Check sheet for the modelled part. Datum: model origin and axes. Units: mm. A direction names the side the tool comes from. Round coordinates to 2 decimals unless told otherwise and drop trailing zeros. Order: outer loops, then holes, each group sorted by start corner. A loop starts at its lowest first (then second) coordinate and runs counter-clockwise, first axis right, second up.
```python
from build123d import *

# Parameters (mm, degrees)
SKETCH1_W           = 5
SKETCH1_H           = 3.7
BOSS_EXTRUDE1_DEPTH = 400
SKETCH2_R           = 1.75
CUT_EXTRUDE1_DEPTH  = 2
SKETCH3_R           = 1
CUT_EXTRUDE2_DEPTH  = 401.036248358
CUT_EXTRUDE3_DEPTH  = 401.048359577
SKETCH5_W           = 10.325646163
SKETCH5_H           = 6.55225139
CUT_EXTRUDE4_DEPTH  = 200


with BuildPart() as part:
    # Sketch1 → Boss-Extrude1 (new body)
    with BuildSketch(Plane.XY):
        with Locations((2.5, 1.85)):
            Rectangle(SKETCH1_W, SKETCH1_H)
    extrude(amount=-BOSS_EXTRUDE1_DEPTH)

    # Sketch2 → Cut-Extrude1 (cut)
    with BuildSketch(Plane(origin=(0, 3.7, 0), x_dir=(1, 0, 0), z_dir=(0, 1, 0))):
        with Locations(Location((2.5, 5, 0), (0, 0, 270))):
            Circle(SKETCH2_R)
        with Locations(Location((2.5, 20, 0), (0, 0, 270))):
            Circle(SKETCH2_R)
        with Locations(Location((2.5, 35, 0), (0, 0, 270))):
            Circle(SKETCH2_R)
        with Locations(Location((2.5, 50, 0), (0, 0, 270))):
            Circle(SKETCH2_R)
        with Locations(Location((2.5, 65, 0), (0, 0, 270))):
            Circle(SKETCH2_R)
        with Locations(Location((2.5, 80, 0), (0, 0, 270))):
            Circle(SKETCH2_R)
        with Locations(Location((2.5, 95, 0), (0, 0, 270))):
            Circle(SKETCH2_R)
        with Locations(Location((2.5, 110, 0), (0, 0, 270))):
            Circle(SKETCH2_R)
        with Locations(Location((2.5, 125, 0), (0, 0, 270))):
            Circle(SKETCH2_R)
        with Locations(Location((2.5, 140, 0), (0, 0, 270))):
            Circle(SKETCH2_R)
        with Locations(Location((2.5, 155, 0), (0, 0, 270))):
            Circle(SKETCH2_R)
        with Locations(Location((2.5, 170, 0), (0, 0, 270))):
            Circle(SKETCH2_R)
        with Locations(Location((2.5, 185, 0), (0, 0, 270))):
            Circle(SKETCH2_R)
        with Locations(Location((2.5, 200, 0), (0, 0, 270))):
            Circle(SKETCH2_R)
        with Locations(Location((2.5, 215, 0), (0, 0, 270))):
            Circle(SKETCH2_R)
        with Locations(Location((2.5, 230, 0), (0, 0, 270))):
            Circle(SKETCH2_R)
        with Locations(Location((2.5, 245, 0), (0, 0, 270))):
            Circle(SKETCH2_R)
        with Locations(Location((2.5, 260, 0), (0, 0, 270))):
            Circle(SKETCH2_R)
        with Locations(Location((2.5, 275, 0), (0, 0, 270))):
            Circle(SKETCH2_R)
        with Locations(Location((2.5, 290, 0), (0, 0, 270))):
            Circle(SKETCH2_R)
        with Locations(Location((2.5, 305, 0), (0, 0, 270))):
            Circle(SKETCH2_R)
        with Locations(Location((2.5, 320, 0), (0, 0, 270))):
            Circle(SKETCH2_R)
        with Locations(Location((2.5, 335, 0), (0, 0, 270))):
            Circle(SKETCH2_R)
        with Locations(Location((2.5, 350, 0), (0, 0, 270))):
            Circle(SKETCH2_R)
        with Locations(Location((2.5, 365, 0), (0, 0, 270))):
            Circle(SKETCH2_R)
        with Locations(Location((2.5, 380, 0), (0, 0, 270))):
            Circle(SKETCH2_R)
        with Locations(Location((2.5, 395, 0), (0, 0, 270))):
            Circle(SKETCH2_R)
    extrude(amount=-CUT_EXTRUDE1_DEPTH, mode=Mode.SUBTRACT)

    # Sketch3 → Cut-Extrude2 (cut, through all)
    with BuildSketch(Plane(origin=(0, 1.7, 0), x_dir=(1, 0, 0), z_dir=(0, 1, 0))):
        with Locations(Location((2.5, 5, 0), (0, 0, 270))):
            Circle(SKETCH3_R)
        with Locations(Location((2.5, 20, 0), (0, 0, 270))):
            Circle(SKETCH3_R)
        with Locations(Location((2.5, 35, 0), (0, 0, 270))):
            Circle(SKETCH3_R)
        with Locations(Location((2.5, 50, 0), (0, 0, 270))):
            Circle(SKETCH3_R)
        with Locations(Location((2.5, 65, 0), (0, 0, 270))):
            Circle(SKETCH3_R)
        with Locations(Location((2.5, 80, 0), (0, 0, 270))):
            Circle(SKETCH3_R)
        with Locations(Location((2.5, 95, 0), (0, 0, 270))):
            Circle(SKETCH3_R)
        with Locations(Location((2.5, 110, 0), (0, 0, 270))):
            Circle(SKETCH3_R)
        with Locations(Location((2.5, 125, 0), (0, 0, 270))):
            Circle(SKETCH3_R)
        with Locations(Location((2.5, 140, 0), (0, 0, 270))):
            Circle(SKETCH3_R)
        with Locations(Location((2.5, 155, 0), (0, 0, 270))):
            Circle(SKETCH3_R)
        with Locations(Location((2.5, 170, 0), (0, 0, 270))):
            Circle(SKETCH3_R)
        with Locations(Location((2.5, 185, 0), (0, 0, 270))):
            Circle(SKETCH3_R)
        with Locations(Location((2.5, 200, 0), (0, 0, 270))):
            Circle(SKETCH3_R)
        with Locations(Location((2.5, 215, 0), (0, 0, 270))):
            Circle(SKETCH3_R)
        with Locations(Location((2.5, 230, 0), (0, 0, 270))):
            Circle(SKETCH3_R)
        with Locations(Location((2.5, 245, 0), (0, 0, 270))):
            Circle(SKETCH3_R)
        with Locations(Location((2.5, 260, 0), (0, 0, 270))):
            Circle(SKETCH3_R)
        with Locations(Location((2.5, 275, 0), (0, 0, 270))):
            Circle(SKETCH3_R)
        with Locations(Location((2.5, 290, 0), (0, 0, 270))):
            Circle(SKETCH3_R)
        with Locations(Location((2.5, 305, 0), (0, 0, 270))):
            Circle(SKETCH3_R)
        with Locations(Location((2.5, 320, 0), (0, 0, 270))):
            Circle(SKETCH3_R)
        with Locations(Location((2.5, 335, 0), (0, 0, 270))):
            Circle(SKETCH3_R)
        with Locations(Location((2.5, 350, 0), (0, 0, 270))):
            Circle(SKETCH3_R)
        with Locations(Location((2.5, 365, 0), (0, 0, 270))):
            Circle(SKETCH3_R)
        with Locations(Location((2.5, 380, 0), (0, 0, 270))):
            Circle(SKETCH3_R)
        with Locations(Location((2.5, 395, 0), (0, 0, 270))):
            Circle(SKETCH3_R)
    extrude(amount=-CUT_EXTRUDE2_DEPTH, mode=Mode.SUBTRACT)

    # Sketch4 → Cut-Extrude3 (cut, through all)
    with BuildSketch(Plane.XY):
        Polygon((0, 2.7), (0.5, 2.2), (0, 1.7), align=None)
        Polygon((5, 2.7), (4.5, 2.2), (5, 1.7), align=None)
    extrude(amount=-CUT_EXTRUDE3_DEPTH, mode=Mode.SUBTRACT)

    # Sketch5 → Cut-Extrude4 (cut)
    with BuildSketch(Plane(origin=(0, 0, -400), x_dir=(-1, 0, 0), z_dir=(0, 0, -1))):
        with Locations((-2.428078688, 2.315270048)):
            Rectangle(SKETCH5_W, SKETCH5_H)
    extrude(amount=-CUT_EXTRUDE4_DEPTH, mode=Mode.SUBTRACT)


solid = part.part
```
Item 1: Scan lines: line 1 along Y through (x, z) = (0.25, -176.5); line 2 along X through (y, z) = (2.2, -104); line 3 along X through (y, z) = (2.3, -50). Record each from-to range of solid material in increasing order.
Answer:
line 1: y = 0 to 1.95, 2.45 to 3.7
line 2: x = 0.5 to 4.5
line 3: x = 0.4 to 0.75, 4.25 to 4.6
Item 2: Sectioned sample at B-B (z = -14). Record the cut outline in (x, y).
Answer:
outline: (0, 0) - (5, 0) - (5, 1.7) - (4.5, 2.2) - (5, 2.7) - (5, 3.7) - (0, 3.7) - (0, 2.7) - (0.5, 2.2) - (0, 1.7) - close
Item 3: Sectioned sample at A-A (x = 2.5). State how many separate pieces and enclosed holes the cut face has, and give its area (3 significant figures).
Answer:
separate pieces: 14
enclosed holes: 0
area: 600 mm2
Item 4: Release check for a two-part mould opening along X. For faces 1 (the flat face through (2, 2, 0)), 2 (the flat face through (1, 1.7, -110)) record: released by +X, released by -X, zero draft, split by the parting line, or undercut.
Answer:
face 1: zero draft
face 2: undercut
Item 5: Access from +Z, -Z, +X, -X, +Y, -Y to the whole of each face (thin tool, end or side, straight path). Record for faces 3 (the flat face through (2, 0, -99)), 4 (the flat face through (1, 1.7, -5)).
Answer:
face 3: +Z, -Z, +X, -X, -Y
face 4: +Y
Item 6: Go/stop test with a flat-tipped pin: P1, Ø1.8, axis at x = 2.5, z = -65.5, coming from the +Y side. Record where the tip stops, or that it passes through.
Answer:
P1: stops at y = 1.7
